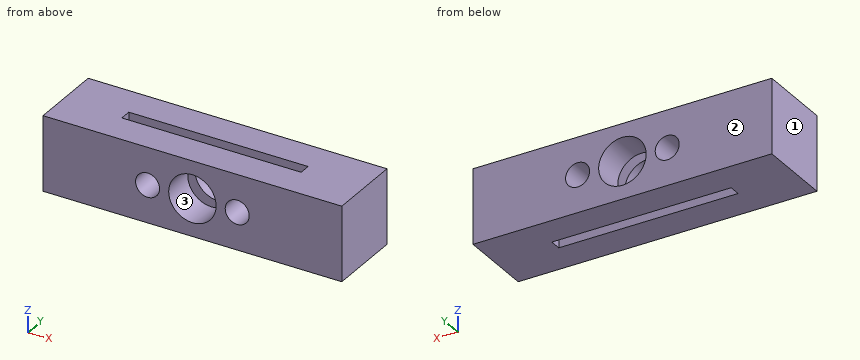
```python
from build123d import *

# Parameters (mm, degrees)
SKETCH1_W               = 63.5
SKETCH1_H               = 15.875
SKETCH1_W_2             = 38.1
SKETCH1_H_2             = 2.446333072
BOSS_EXTRUDE1_DEPTH     = 7.9375
F_1_4_20_TAPPED_HOLE1_D = 5.1054
F_3_8_CLEARANCE_HOLE1_D = 10.0838


with BuildPart() as part:
    # Sketch1 → Boss-Extrude1 (new, symmetric)
    with BuildSketch(Plane.XY):
        Rectangle(SKETCH1_W, SKETCH1_H)
        Rectangle(SKETCH1_W_2, SKETCH1_H_2, mode=Mode.SUBTRACT)
    extrude(amount=BOSS_EXTRUDE1_DEPTH, both=True)

    # 1/4-20 Tapped Hole1 (through all)
    with Locations(Plane(origin=(0, 7.9375, 0), x_dir=(1, 0, 0), z_dir=(0, 1, 0))):
        with Locations((9.525, 0), (-9.525, 0)):
            Hole(F_1_4_20_TAPPED_HOLE1_D / 2)

    # 3/8 Clearance Hole1 (through all)
    with Locations(Plane(origin=(0, 7.9375, 0), x_dir=(1, 0, 0), z_dir=(0, 1, 0))):
        with Locations((0, 0)):
            Hole(F_3_8_CLEARANCE_HOLE1_D / 2)


solid = part.part
```
Work out the finished part from the listing and answer in its coordinate system (mm). Face numbers are marked on the shaded views. Round coordinates to 2 decimals unless told otherwise and drop trailing zeros. Loops run counter-clockwise (first coordinate to the right, second up) from the corner with the lowest first, then second, coordinate; pieces in that order, holes last. Notation, with made-up numbers: M 64.5,-11.5 L 69.5,-11.5 A24 ccw 69.5,6.5 Z; hole C 63,14.25 d7. An arc over 180 degrees is marked long. Use CSV: the item, a comma, the result in double quotes.
Q1. This flat-tipped pin is pushed along its axis until it touches: pin 1 (4 mm diameter, centred on x = -9.525, z = 0, fed in from -Y). Where does it stop, or does it pass through?
Determined:
pin 1,"through"
Q2. The mould has two halves that part along X. Classify the marked faces 1, 2 and 3: pulls with the +X half, pulls with the -X half, needs draft (parallel to the pull), parting line crosses it, or undercut.
Determined:
face 1,"pulls with the -X half"
face 2,"needs draft"
face 3,"undercut"
Q3. Section B-B, the plane y = -4.25 is taken. State how many separate pieces and enclosed holes the cut face has, then the cut area to 3 significant figures.
Determined:
separate pieces,"1"
enclosed holes,"3"
area,"887 mm2"
Q4. Consider L1, parallel to Y at x = 6.5, z = -6.25; L2, parallel to Z at x = 0, y = 3; L3, parallel to X at y = 6.5, z = -2.25. Determine where each line is inside the solid, lowest interval first.
Determined:
L1,"-7.94 to -1.22, 1.22 to 7.94"
L2,"-7.94 to -5.04, 5.04 to 7.94"
L3,"-31.75 to -10.73, -8.32 to -4.51, 4.51 to 8.32, 10.73 to 31.75"
Q5. Section A-A, the plane x = 0 is taken. Determine the outline of the cut face in (y, z), then the cut area to 3 significant figures.
Determined:
outline,"M -7.94,-7.94 L -1.22,-7.94 L -1.22,-5.04 L -7.94,-5.04 Z; M -7.94,5.04 L -1.22,5.04 L -1.22,7.94 L -7.94,7.94 Z; M 1.22,-7.94 L 7.94,-7.94 L 7.94,-5.04 L 1.22,-5.04 Z; M 1.22,5.04 L 7.94,5.04 L 7.94,7.94 L 1.22,7.94 Z"
area,"77.8 mm2"
Q6. Section D-D, the plane z = 6.5 is taken. Determine the outline of the cut face in (x, y).
Determined:
outline,"M -31.75,-7.94 L 31.75,-7.94 L 31.75,7.94 L -31.75,7.94 Z; hole M -19.05,-1.22 L 19.05,-1.22 L 19.05,1.22 L -19.05,1.22 Z"
